CAD build for the part. Positions are in the model's coordinates, mm. Face numbers are marked on the shaded views. A direction names the side the tool comes from. Give positions to 0.01 mm unless a question says otherwise; leave off trailing zeros. Order: outer loops, then holes, each group sorted by start corner. A loop starts at its lowest first (then second) coordinate and runs counter-clockwise, first axis right, second up.
Item 1: Flat gauge pins, fed straight in: P1, Ø1.5, axis at y = 25, z = 1.5, coming from the -X side; P2, Ø3.5, axis at x = 1, y = 23, coming from the -Z side. Where does each tip first touch, or does it go through?
Item 2: Two-plate mould, pull along X, no slides. Class the marked faces 1, 2 and 3: released by +X, released by -X, zero draft, split by the parting line, or undercut.
Item 3: Band-saw the part on B-B on y = 58. Give the cut face in (x, z), plus the area to 3 significant figures.
Item 4: Wall check: L1, parallel to Y at x = 95.5, z = 53; L2, parallel to X at y = 56, z = 69.5; L3, parallel to Z at x = 43, y = 120. Give the ranges that are in metal, low to high.
Item 5: Band-saw the part on A-A on x = 42. Give the cut face in (y, z), plus the area to 3 significant figures.
Item 6: Band-saw the part on C-C on z = 45. Give the cut face in (x, y), plus the area to 3 significant figures.
Item 7: Which spindle directions (+Z, -Z, +X, -X, +Y, -Y) get a long thin tool onto all of the face, cutting with end or side? Do the marked faces 4 and 5. Say none if no direction does.
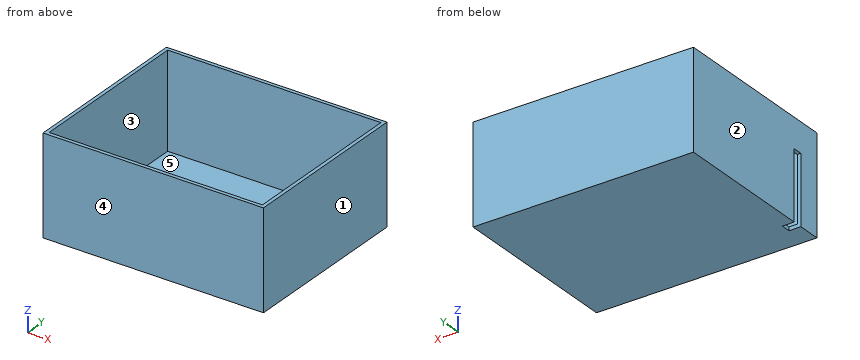
```python
from build123d import *

# Parameters (mm, degrees)
SKETCH_1_W                      = 186
SKETCH_1_H                      = 149
FLOOR_T3_DEPTH                  = 3
SKETCH_2_W                      = 186
SKETCH_2_H                      = 149
SKETCH_2_W_2                    = 180
SKETCH_2_H_2                    = 143
WALLS_T3_DEPTH80_DEPTH          = 83
SKETCH_3_W                      = 11
SKETCH_3_H                      = 8
SERVO_STAND_RELIEF_W8_H58_DEPTH = 58


with BuildPart() as part:
    # 草图1 → Floor_T3 (new body)
    with BuildSketch(Plane.XY):
        with Locations((93, 74.5)):
            Rectangle(SKETCH_1_W, SKETCH_1_H)
    extrude(amount=FLOOR_T3_DEPTH)

    # 草图2 → Walls_T3_depth80 (add)
    with BuildSketch(Plane.XY):
        with Locations((93, 74.5)):
            Rectangle(SKETCH_2_W, SKETCH_2_H)
        with Locations((93, 74.5)):
            Rectangle(SKETCH_2_W_2, SKETCH_2_H_2, mode=Mode.SUBTRACT)
    extrude(amount=WALLS_T3_DEPTH80_DEPTH)

    # 草图3 → Servo_stand_relief_W8_H58 (cut)
    with BuildSketch(Plane.XY):
        with Locations((4.5, 23.5)):
            Rectangle(SKETCH_3_W, SKETCH_3_H)
    extrude(amount=SERVO_STAND_RELIEF_W8_H58_DEPTH, mode=Mode.SUBTRACT)


solid = part.part
```
The answers:
1. P1: stops at x = 10
1. P2: stops at z = 58
2. face 1: released by +X
2. face 2: released by -X
2. face 3: undercut
3. outline: (0, 0) - (186, 0) - (186, 83) - (183, 83) - (183, 3) - (3, 3) - (3, 83) - (0, 83) - close
3. area: 1,040 mm2
4. L1: y = 0 to 3, 146 to 149
4. L2: x = 0 to 3, 183 to 186
4. L3: z = 0 to 3
5. outline: (0, 0) - (149, 0) - (149, 83) - (146, 83) - (146, 3) - (3, 3) - (3, 83) - (0, 83) - close
5. area: 927 mm2
6. outline: (0, 0) - (186, 0) - (186, 149) - (0, 149) - (0, 27.5) - (3, 27.5) - (3, 146) - (183, 146) - (183, 3) - (3, 3) - (3, 19.5) - (0, 19.5) - close
6. area: 1,950 mm2
7. face 4: +Z, -Z, +X, -X, -Y
7. face 5: +Z
